CAD build for the part. Positions are in the model's coordinates, mm. A direction names the side the tool comes from. Coordinates: 2 decimals unless noted, no trailing zeros. Order: outer loops, then holes, each group sorted by start corner. A loop starts at its lowest first (then second) coordinate and runs counter-clockwise, first axis right, second up. Notation, with made-up numbers: M 10,14.5 L 30,14.5 A22 cw 30,45.5 Z; hole C 17,24.5 d7. An arc over 180 degrees is marked long. Write item = value, one per line.
Autodesk Inventor part; units mm, degrees
ref_plane "YZ Plane" through (0, 0, 0) normal (1, 0, 0) x (0, 1, 0)
ref_plane "XZ Plane" through (0, 0, 0) normal (0, 1, 0) x (-1, 0, 0)
ref_plane "XY Plane" through (0, 0, 0) normal (0, 0, 1) x (1, 0, 0)
sketch "Esboço1" plane through (0, 0, 0) normal (0, 1, 0) x (-1, 0, 0)
  line L0 (-1.2, -1.2) -> (-37.2, -1.2)
  line L1 (-1.2, -19.2) -> (-1.2, -1.2)
  arc A0 (-37.2, -1.2) -> (-37.2, -19.2) centre (-37.2, -10.2) ccw
  line L2 (-1.2, -19.2) -> (-37.2, -19.2)
  line L3 (-37.2, -20.4) -> (0, -20.4)
  line L4 (0, -20.4) -> (0, 0)
  line L5 (0, 0) -> (-37.2, 0)
  arc A1 (-37.2, 0) -> (-37.2, -20.4) centre (-37.2, -10.2) ccw
  line L6 (-1.2, -1.2) -> (0, -1.2)
  line L7 (-1.2, -19.2) -> (0, -19.2)
  point P0 (-1.2, -10.2)
  dimension "d0" = 18
  dimension "d3" = 18
  dimension "d5" = 36
  dimension "d6" = 1.2
extrude "Extrusão1" add sketch "Esboço1" against normal blind 1.2
extrude "Extrusão2" add sketch "Esboço1" along normal blind 20 contours L0 A0 L2 L7 L4 L3 A1 L5 L6
fillet "Arredondamento1" radius 9 3 edges at (46.2, 0, -10.2) (18.6, 0, -1.2) (18.6, 0, -19.2)
sketch "Esboço2" plane through (0, -1.2, 0) normal (0, 0, 1) x (1, 0, 0)
  line L0 (37.2, 21.2) -> (46.2, 21.2)
  line L1 (37.2, 0) -> (0, 0)
  line L2 (37.2, 1.2) -> (37.2, 21.2)
  line L3 (0, 21.2) -> (0, 0)
  line L4 (47.4, 21.2) -> (37.2, 21.2)
  line L5 (0, 9) -> (37.2, 21.2)
  line L6 (37.2, 21.2) -> (0, 21.2)
  line L7 (0, 21.2) -> (37.2, 21.2)
  line L8 (37.2, 21.2) -> (47.4, 19.4015)
  line L9 (47.4, 21.2) -> (47.4, 0)
  line L10 (37.2, 21.2) -> (47.5574, 21.2) construction
  line L11 (47.4, 19.4015) -> (47.4, 21.2)
  line L12 (47.4, 21.2) -> (47.4, 0)
  line L13 (37.2, 21.2) -> (47.4, 21.2)
  line L14 (0, 9) -> (0, 21.2)
  point P0 (0, 1.2)
  point P1 (0, 10.6)
  point P2 (0, 10.6)
  dimension "d13" = 9
  dimension "d16" = 10
extrude "Extrusão3" cut sketch "Esboço2" against normal up to surface (20.4 mm away)
equation "\"d0\" = Diâmetro_esfera"
equation "\"d3\" = Diâmetro_esfera"
equation "\"d5\" = 2 * Diâmetro_esfera"
equation "\"d6\" = Margem"
equation "\"d7\" = Margem"
equation "\"d11\" = 0.5 * Diâmetro_esfera"
equation "\"d13\" = 0.5 * Diâmetro_esfera"
equation "\"Diâmetro_esfera\" = 18"
equation "\"Filamento\" = 0.4"
equation "\"Margem\" = 3 * Filamento"
equation "\"Parafuso\" = 3"
properties part number "Receptor pequeno" material "Plástico PET"
(1) Pin check, flat tips, straight feed: pin 1 Ø8 at (x, z) = (40, -7.5) entering from +Y; pin 2 Ø3 at (y, z) = (16, -12) entering from +X; pin 3 Ø1 at (x, z) = (37, -7) entering from +Y. Stop position of each tip, or through.
Evaluation:
pin_1 = 4.67
pin_2 = 47.4
pin_3 = 0.8
(2) Slice it at D-D, the plane y = 14. Write the cut outline in (x, z).
Evaluation:
outline = M 18.9,-20.4 L 37.2,-20.4 A10.2 ccw 37.2,0 L 18.9,0 L 18.9,-1.2 L 37.2,-1.2 A9 cw 37.2,-19.2 L 18.9,-19.2 Z
(3) Slice it at B-B, the plane y = 17.25. Write the cut outline in (x, z), then the cut area to 3 significant figures.
Evaluation:
outline = M 28.81,-20.4 L 37.2,-20.4 A10.2 ccw 37.2,0 L 28.81,0 L 28.81,-1.2 L 37.2,-1.2 A9 cw 37.2,-19.2 L 28.81,-19.2 Z
area = 56.3 mm²
(4) Wall check: line 1 (Z direction, x = 29, y = 9.5); line 2 (Z direction, x = 43, y = 17.75); line 3 (X direction, y = 15.5, z = -10.25). Give the ranges that are in metal, low to high. Write a range as from..to.
Evaluation:
line_1 = -20.4..-19.2, -1.2..0
line_2 = -18.59..-17.08, -3.32..-1.81
line_3 = 46.2..47.4
(5) Pull direction Z, two halves, no side cores. Call faces 3 (the face through (47.4, 9.3, -10.4)), 4 (the face through (18.34, 2.706, -16.634)), 5 (the face through (22, 7, 0)): +Z half, -Z half, draft (parallel to the pull), parting line (faces both ways), or undercut.
Evaluation:
face_3 = parting line
face_4 = undercut
face_5 = +Z half
(6) Tool access for faces 1 (the face through (24, 13, -1.2)), 2 (the face through (18.3, 13.8, -0.6)): list every direction of +Z, -Z, +X, -X, +Y, -Y with a clear straight run to the whole face (end or side of a thin tool).
Evaluation:
face_1 = -X, +Y
face_2 = +Z, -Z, -X, +Y
